```python
from build123d import *

# Parameters (mm, degrees)
F0_W     = 71
F0_H     = 7.4
F0_R     = 3
F1_DEPTH = 3.95
F0_R_2   = 2.499
F2_DEPTH = 3.45
F3_R     = 3.69999


# Not quite as in the source:
# - a fillet or chamfer is up to 0.001 mm smaller than in the source, because OpenCascade refuses the exact size


with BuildPart() as f1:
    # F0 (on Front) → F1 (new body, symmetric)
    with BuildSketch(Plane.XZ):
        Rectangle(F0_W, F0_H)
        with Locations((-32, 0)):
            Circle(F0_R, mode=Mode.SUBTRACT)
        with Locations((-24, 0)):
            Circle(F0_R, mode=Mode.SUBTRACT)
        with Locations((-16, 0)):
            Circle(F0_R, mode=Mode.SUBTRACT)
        with Locations((-8, 0)):
            Circle(F0_R, mode=Mode.SUBTRACT)
        Circle(F0_R, mode=Mode.SUBTRACT)
        with Locations((8, 0)):
            Circle(F0_R, mode=Mode.SUBTRACT)
        with Locations((16, 0)):
            Circle(F0_R, mode=Mode.SUBTRACT)
        with Locations((24, 0)):
            Circle(F0_R, mode=Mode.SUBTRACT)
        with Locations((32, 0)):
            Circle(F0_R, mode=Mode.SUBTRACT)
    extrude(amount=F1_DEPTH, both=True)

    # F0 (on Front) → F2 (join, symmetric)
    with BuildSketch(Plane.XZ):
        with Locations((-32, 0)):
            Circle(F0_R)
        with Locations((-32, 0)):
            Circle(F0_R_2, mode=Mode.SUBTRACT)
        with Locations((-24, 0)):
            Circle(F0_R)
        with Locations((-24, 0)):
            Circle(F0_R_2, mode=Mode.SUBTRACT)
        with Locations((-16, 0)):
            Circle(F0_R)
        with Locations((-16, 0)):
            Circle(F0_R_2, mode=Mode.SUBTRACT)
        with Locations((-8, 0)):
            Circle(F0_R)
        with Locations((-8, 0)):
            Circle(F0_R_2, mode=Mode.SUBTRACT)
        Circle(F0_R)
        Circle(F0_R_2, mode=Mode.SUBTRACT)
        with Locations((8, 0)):
            Circle(F0_R)
        with Locations((8, 0)):
            Circle(F0_R_2, mode=Mode.SUBTRACT)
        with Locations((16, 0)):
            Circle(F0_R)
        with Locations((16, 0)):
            Circle(F0_R_2, mode=Mode.SUBTRACT)
        with Locations((24, 0)):
            Circle(F0_R)
        with Locations((24, 0)):
            Circle(F0_R_2, mode=Mode.SUBTRACT)
        with Locations((32, 0)):
            Circle(F0_R)
        with Locations((32, 0)):
            Circle(F0_R_2, mode=Mode.SUBTRACT)
    extrude(amount=F2_DEPTH, both=True)

    # F3 (radius 3.7 in the source; OpenCascade refuses exactly that, so slightly less here)
    f3_edges = [f1.edges().sort_by_distance(p)[0] for p in [
        (-35.5, 0, 3.7),
        (-35.5, 0, -3.7),
        (35.5, 0, 3.7),
        (35.5, 0, -3.7),
    ]]
    fillet(f3_edges, radius=F3_R)


solid = f1.part
```
Here's how the part is built. I have some questions about the finished solid (model axes, mm). A direction names the side the tool comes from. Round coordinates to 2 decimals unless told otherwise and drop trailing zeros. Order: outer loops, then holes, each group sorted by start corner. A loop starts at its lowest first (then second) coordinate and runs counter-clockwise, first axis right, second up. Notation, with made-up numbers: (-2, 53.25) -> (44, 53.25) arc R37 cw to (44, 92.25) -> close; hole circle Ø1 at (50, -31.5). An arc over 180 degrees is marked (long way). Use a Markdown table: item, result. Add a question column.
(1) If we mould it in two halves opening along X, with no side actions, what happens to faces 1 (the face through (-34.44, 0.06, 2.59)), 2 (the face through (34.39, -0.06, -2.64)), 3 (the face through (-19, -3.7, 0.1))? For each: released by +X, released by -X, zero draft, split by the parting line, or undercut.
(2) I need wall thicknesses on line 1 along Z through (x, y) = (-8, -1.2); line 2 along Y through (x, z) = (17.5, -2.5); line 3 along Z through (x, y) = (-30.5, 2.25). Which ranges of each line are inside material? Lowest first, please.
(3) Suppose I cut it at B-B, the plane y = 0.75. Count the separate pieces of the cut face and the enclosed holes in it, and give its area (3 significant figures).
(4) Suppose I cut it at D-D, the plane x = 14.5. Please give me the cut outline in (y, z).
(5) For pin 1 Ø1.5 at (y, z) = (-1.5, 1) entering from -X; pin 2 Ø1.8 at (x, z) = (23.5, 0) entering from +Y; pin 3 Ø1 at (y, z) = (2, -3) entering from +X, each with a flat end and sliding along its axis, tell me the tip position at first contact or that it passes through.
(6) Suppose I cut it at A-A, the plane x = -24. Please give me the cut outline in (y, z), and give its area (3 significant figures).
(7) For faces 4 (the face through (-10, 3.45, 2)), 5 (the face through (6, -3.45, 2)), 6 (the face through (34.384, 0.048, 0.751)), which set-ups out of +Z, -Z, +X, -X, +Y, -Y let a thin tool reach every point of the face, with its end or its side?
Verdict:
| question | item | result |
|---|---|---|
| 1 | face 1 | released by -X |
| 1 | face 2 | released by +X |
| 1 | face 3 | undercut |
| 2 | line 1 | -3.7 to -2.5, 2.5 to 3.7 |
| 2 | line 2 | -3.45 to 3.45 |
| 2 | line 3 | -3.7 to -2, 2 to 3.7 |
| 3 | separate pieces | 1 |
| 3 | enclosed holes | 9 |
| 3 | area | 337 mm2 |
| 4 | outline | (-3.95, -3.7) -> (3.95, -3.7) -> (3.95, -2.6) -> (3.45, -2.6) -> (3.45, -2) -> (-3.45, -2) -> (-3.45, -2.6) -> (-3.95, -2.6) -> close; (-3.95, 2.6) -> (-3.45, 2.6) -> (-3.45, 2) -> (3.45, 2) -> (3.45, 2.6) -> (3.95, 2.6) -> (3.95, 3.7) -> (-3.95, 3.7) -> close |
| 5 | pin 1 | x = -35.49 |
| 5 | pin 2 | through |
| 5 | pin 3 | x = 34.53 |
| 6 | outline | (-3.95, -3.7) -> (3.95, -3.7) -> (3.95, -3) -> (3.45, -3) -> (3.45, -2.5) -> (-3.45, -2.5) -> (-3.45, -3) -> (-3.95, -3) -> close; (-3.95, 3) -> (-3.45, 3) -> (-3.45, 2.5) -> (3.45, 2.5) -> (3.45, 3) -> (3.95, 3) -> (3.95, 3.7) -> (-3.95, 3.7) -> close |
| 6 | area | 18.0 mm2 |
| 7 | face 4 | +Y |
| 7 | face 5 | -Y |
| 7 | face 6 | +Y, -Y |
